Read the model definition and answer for the solid it produces. Units are mm, in the model's axes. A direction names the side the tool comes from. Give positions to 0.01 mm unless a question says otherwise; leave off trailing zeros. Order: outer loops, then holes, each group sorted by start corner. A loop starts at its lowest first (then second) coordinate and runs counter-clockwise, first axis right, second up. Notation, with made-up numbers: (21.5, -12) -> (48.5, -12) arc R12 ccw to (48.5, 4) -> close; hole circle Ø6 at (83, 25.25). An arc over 180 degrees is marked (long way). One line per question, with ' | ' between items. Start each with the question number.
```python
from build123d import *

# Parameters (mm, degrees)
SKETCH1_R           = 2.75
BASEHEAD_DEPTH      = 3
SKETCH2_R           = 1.5
BASEBODY_DEPTH      = 12
HEXAGONSOCKET_DEPTH = 1.3
TOPFILLET_R         = 0.375
CHAMFER1_SIZE       = 0.1


with BuildPart() as part:
    # Sketch1 → BaseHead (new body)
    with BuildSketch(Plane(origin=(0, 0, 0), x_dir=(0, 0, -1), z_dir=(1, 0, 0))):
        Circle(SKETCH1_R)
    extrude(amount=BASEHEAD_DEPTH)

    # Sketch2 → BaseBody (add)
    with BuildSketch(Plane(origin=(3, 0, 0), x_dir=(0, 0, -1), z_dir=(1, 0, 0))):
        Circle(SKETCH2_R)
    extrude(amount=BASEBODY_DEPTH)

    # Sketch3 → HexagonSocket (cut)
    with BuildSketch(Plane(origin=(0, 0, 0), x_dir=(0, 0, -1), z_dir=(1, 0, 0))):
        Polygon((1.443375673, 0), (0.721687836, 1.25), (-0.721687836, 1.25), (-1.443375673, 0), (-0.721687836, -1.25), (0.721687836, -1.25), align=None)
    extrude(amount=HEXAGONSOCKET_DEPTH, mode=Mode.SUBTRACT)

    # Sketch4 → Cut-Revolve1 (revolve, cut)
    with BuildSketch(Plane(origin=(-4.19613823, 0.75, 0), x_dir=(-1, 0, 0), z_dir=(0, 0, 1))):
        Polygon((-5.49613823, 2), (-6.217826066, 0.75), (-5.49613823, 0.75), align=None)
    revolve(axis=Axis((0.838992387, 0, 0), (-1, 0, 0)), mode=Mode.SUBTRACT)

    # TopFillet
    topfillet_edges = [part.edges().sort_by_distance(p)[0] for p in [
        (0, 0, 2.75),
    ]]
    fillet(topfillet_edges, radius=TOPFILLET_R)

    # Chamfer1
    chamfer1_edges = [part.edges().sort_by_distance(p)[0] for p in [
        (15, 0, 1.5),
    ]]
    chamfer(chamfer1_edges, length=CHAMFER1_SIZE)


solid = part.part
```
Q1. A cutting plane is placed at A-A, the plane x = 6. Determine the outline of the cut face in (y, z).
Q2. Given P1, Ø1.5, axis at x = 8.5, y = 1, coming from the -Z side; P2, Ø0.6, axis at x = 1, z = -0.5, coming from the -Y side; P3, Ø2, axis at x = 9.5, z = -0.5, coming from the +Y side, each flat-ended and moving along its own axis, determine where each tip first touches the part or whether it passes through.
Q3. Determine the mould class of faces 4 (the flat face through (0.64, 0.63, 1.08)), 5 (the flat face through (15, 0, 0)), 6 (the cylindrical face through (1.669, -2.685, 0.596)), 7 (the flat face through (0.64, -0.63, -1.08)) for opening direction Y: pulls with the +Y half, pulls with the -Y half, needs draft (parallel to the pull), parting line crosses it, or undercut.
Q4. Find the intervals of material crossed by line 1 (X direction, y = -1.65, z = -0.15); line 2 (Z direction, x = 13.75, y = 0.1), in increasing order.
Q5. Which of the six approach directions +Z, -Z, +X, -X, +Y, -Y give full straight-line access (tool end or side, diameter ignored) to faces 1 (the flat face through (0, -2, 0)), 2 (the flat face through (3, -1.2, -1.2)), 3 (the flat face through (1, -1.25, 0))?
Geometry results:
1) outline: circle Ø3 at (0, 0)
2) P1: z = -1.48 | P2: y = -2.74 | P3: y = 1.5
3) face 4: undercut | face 5: needs draft | face 6: parting line crosses it | face 7: undercut
4) line 1: 0 to 3 | line 2: -1.5 to 1.5
5) face 1: +Z, -Z, -X, +Y, -Y | face 2: +X | face 3: -X
